```python
from build123d import *

# Parameters (mm, degrees)
SKETCH_R           = 19
PAD_DEPTH          = 34
SKETCH001_R        = 19
PAD001_DEPTH       = 1
SKETCH002_R        = 10
PAD002_DEPTH       = 5
SKETCH003_R        = 3
PAD003_DEPTH       = 13
SKETCH004_W        = 5
SKETCH004_H        = 3
POCKET_DEPTH       = 10
SKETCH005_R        = 1.5
POCKET001_DEPTH    = 8
POLARPATTERN_COUNT = 3


with BuildPart() as part:
    # Sketch → Pad (new body)
    with BuildSketch(Plane.XZ):
        Circle(SKETCH_R)
    extrude(amount=PAD_DEPTH)

    # Sketch001 (on Face3 of Pad) → Pad001 (join)
    with BuildSketch(Plane.XZ.offset(34)):
        Circle(SKETCH001_R)
    extrude(amount=PAD001_DEPTH)

    # Sketch002 (on Face4 of Pad001) → Pad002 (join)
    with BuildSketch(Plane.XZ.offset(35)):
        Circle(SKETCH002_R)
    extrude(amount=PAD002_DEPTH)

    # Sketch003 (on Face6 of Pad002) → Pad003 (join)
    with BuildSketch(Plane.XZ.offset(40)):
        Circle(SKETCH003_R)
    extrude(amount=PAD003_DEPTH)

    # Sketch004 (on Face8 of Pad003) → Pocket (cut)
    with BuildSketch(Plane.XZ.offset(53)):
        with Locations((0, 3.8)):
            Rectangle(SKETCH004_W, SKETCH004_H)
    extrude(amount=-POCKET_DEPTH, mode=Mode.SUBTRACT)

    # Sketch005 (on Face4 of Pad001) → Pocket001 (cut)
    with BuildSketch(Plane.XZ.offset(35)):
        with Locations((0, 14)):
            Circle(SKETCH005_R)
        with Locations((7.5, 12.990381)):
            Circle(SKETCH005_R)
    pocket001 = extrude(amount=-POCKET001_DEPTH, mode=Mode.SUBTRACT)

    # PolarPattern: Pocket001 ×3 about axis
    polarpattern_axis = Axis((0, -35, 0), (0, -1, 0))
    for i in range(1, POLARPATTERN_COUNT):
        add(pocket001.rotate(polarpattern_axis, i * 360 / POLARPATTERN_COUNT), mode=Mode.SUBTRACT)


solid = part.part
```
The model under review builds one solid part; all positions refer to its coordinate system, in mm. A direction names the side the tool comes from. Round coordinates to 2 decimals unless told otherwise and drop trailing zeros. Loops run counter-clockwise (first coordinate to the right, second up) from the corner with the lowest first, then second, coordinate; pieces in that order, holes last. Notation, with made-up numbers: M 3.25,-25 L 56.25,-25 A6 ccw 56.25,-18 Z; hole C 75.25,69.25 d9. An arc over 180 degrees is marked long. Write item = value, one per line.
Item 1: For line 1 (X direction, y = -31.5, z = -6.5); line 2 (Y direction, x = 12, z = 10); line 3 (Z direction, x = -0.5, y = -24), list the stretches that pass through material, from the lowest coordinate up. Write a range as [from, to].
Return value:
line_1 = [-17.85, -13.54], [-10.71, 10.71], [13.54, 17.85]
line_2 = [-35, 0]
line_3 = [-18.99, 18.99]
Item 2: Insertion check: P1, Ø4, axis at x = 10.5, z = -13.5, coming from the +Y side; P2, Ø5, axis at y = -17.5, z = 14.5, coming from the -X side; P3, Ø5, axis at y = -18, z = 13.5, coming from the +X side; P4, Ø1.5, axis at x = 9.5, z = -12, coming from the -Y side. Each pin has a flat end and moves straight along its axis. Give the tip position at first contact, or say it passes through.
Return value:
P1 = 0
P2 = -14.73
P3 = 15.49
P4 = -35
Item 3: Take a section at B-B on z = 0. Write out the cut boundary in (x, y).
Return value:
outline = M -19,-35 L -16.5,-35 L -16.5,-27 L -13.5,-27 L -13.5,-35 L -10,-35 L -10,-40 L -3,-40 L -3,-53 L 3,-53 L 3,-40 L 10,-40 L 10,-35 L 19,-35 L 19,0 L -19,0 Z
Item 4: The part is to be moulded in two halves that separate along X. For faces 4 (the cylindrical face through (-2.17, -37.47, -9.76)), 5 (the flat face through (0, -53, 0)), 6 (the flat face through (8, -27, -13)), say which applies: released by +X, released by -X, zero draft, split by the parting line, or undercut.
Return value:
face_4 = split by the parting line
face_5 = zero draft
face_6 = undercut
Item 5: Take a section at A-A on x = 0. Write out the cut boundary in (y, z).
Return value:
outline = M -53,-3 L -40,-3 L -40,-10 L -35,-10 L -35,-19 L 0,-19 L 0,19 L -35,19 L -35,15.5 L -27,15.5 L -27,12.5 L -35,12.5 L -35,10 L -40,10 L -40,3 L -43,3 L -43,2.3 L -53,2.3 Z
Item 6: Machinability: for faces 1 (the flat face through (0, -48, 2.3)), 2 (the flat face through (0, 0, 0)), 3 (the flat face through (2.1, -40, 2.4)), which of the approach directions +Z, -Z, +X, -X, +Y, -Y give a long, thin tool a straight path to every point of the face, cutting with its end or side? Answer none if there is none.
Return value:
face_1 = +Z, +X, -X, -Y
face_2 = +Z, -Z, +X, -X, +Y
face_3 = -Y
Item 7: Take a section at D-D on x = -9. Write out the cut boundary in (y, z).
Return value:
outline = M -40,-4.36 L -35,-4.36 L -35,-16.73 L 0,-16.73 L 0,16.73 L -35,16.73 L -35,4.36 L -40,4.36 Z
Item 8: Take a section at C-C on x = -15. Write out the cut boundary in (y, z).
Return value:
outline = M -35,-11.66 L 0,-11.66 L 0,11.66 L -35,11.66 L -35,1.5 L -27,1.5 L -27,-1.5 L -35,-1.5 Z
